from build123d import *

# Parameters (mm, degrees)
ESQUISSE1_R        = 3.5
ESQUISSE1_R_2      = 1.45
BOSS_EXTRU_1_DEPTH = 5


with BuildPart() as part:
    # Esquisse1 → Boss.-Extru.1 (new body)
    with BuildSketch(Plane.XY):
        with BuildLine():
            Line((-23.520309347, 11.085383373), (-24.358908183, 11.706502475))
            ThreePointArc((-24.358908183, 11.706502475), (-24.845678879, 12.118284674), (-25.260449538, 12.602511471))
            ThreePointArc((-25.260449538, 12.602511471), (-32.357200459, 11.85890316), (-28.166092976, 6.083832163))
            ThreePointArc((-28.166092976, 6.083832163), (-26.925251175, 6.018420638), (-25.765053202, 5.573552451))
            ThreePointArc((-25.765053202, 5.573552451), (-23.38866031, 3.221956107), (-22.477205459, 0.005358743))
            ThreePointArc((-22.477205459, 0.005358743), (-22.840333933, -2.118823087), (-23.958742219, -3.960879992))
            ThreePointArc((-23.958742219, -3.960879992), (-24.504417424, -4.651802838), (-24.955377519, -5.407958113))
            ThreePointArc((-24.955377519, -5.407958113), (-25.122929262, -5.539522919), (-25.331723523, -5.497240048))
            add(Edge.make_bspline(
                [(-27.707778762, -5.50497209), (-27.463755153, -5.421858651), (-27.208964141, -5.35321212), (-26.847281922, -5.290646334), (-26.755999287, -5.277514723), (-26.472348923, -5.247412771), (-26.276940328, -5.237520804), (-25.988433148, -5.260972525), (-25.921846007, -5.267964485), (-25.794475247, -5.289589568), (-25.737903956, -5.299827616), (-25.600175401, -5.340785914), (-25.51525962, -5.375688947), (-25.386655187, -5.458237644), (-25.359770306, -5.476681289), (-25.331723523, -5.497240048)],
                knots=[0, 0, 0, 0, 0.401379624, 0.401379624, 0.532597126, 0.532597126, 0.795032129, 0.795032129, 0.872293172, 0.872293172, 0.929035383, 0.929035383, 0.985777595, 0.985777595, 1, 1, 1, 1], degree=3))
            ThreePointArc((-27.707778762, -5.50497209), (-27.801973044, -5.564338041), (-27.859240924, -5.659822431))
            ThreePointArc((-27.859240924, -5.659822431), (-27.97528469, -6.057416591), (-28.073587363, -6.459764521))
            ThreePointArc((-28.073587363, -6.459764521), (-28.071734795, -6.57109038), (-28.019843727, -6.669600257))
            add(Edge.make_bspline(
                [(-25.965992802, -7.864336487), (-26.163909603, -7.885982848), (-26.294618647, -7.863685821), (-26.490123672, -7.810689646), (-26.569333075, -7.776803309), (-26.723621302, -7.70842793), (-26.794279204, -7.672573545), (-27.014611477, -7.551431096), (-27.148381506, -7.461400071), (-27.399282552, -7.274477346), (-27.514428456, -7.1774816), (-27.765918403, -6.946352168), (-27.896967937, -6.810004535), (-28.019843727, -6.669600257)],
                knots=[0, 0, 0, 0, 0.081187854, 0.081187854, 0.177126147, 0.177126147, 0.27306444, 0.27306444, 0.491378598, 0.491378598, 0.709692757, 0.709692757, 1, 1, 1, 1], degree=3))
            ThreePointArc((-25.965992802, -7.864336487), (-25.764030643, -7.932116803), (-25.68471018, -8.12983162))
            ThreePointArc((-25.68471018, -8.12983162), (-25.693544809, -8.474793397), (-25.684712274, -8.819755228))
            ThreePointArc((-25.684712274, -8.819755228), (-25.764033937, -9.017469563), (-25.965996507, -9.085248653))
            add(Edge.make_bspline(
                [(-28.019854683, -10.279972417), (-27.850080758, -10.085982263), (-27.663748533, -9.899137116), (-27.381805435, -9.664112445), (-27.309318159, -9.607098819), (-27.078720715, -9.439204582), (-26.914437891, -9.332933591), (-26.652857483, -9.208989788), (-26.591695348, -9.181751432), (-26.470576489, -9.136793922), (-26.416465288, -9.117374686), (-26.2767097, -9.083981334), (-26.185718951, -9.071750358), (-26.033069896, -9.078937415), (-26.000565097, -9.081467639), (-25.965996507, -9.085248653)],
                knots=[0, 0, 0, 0, 0.401379627, 0.401379627, 0.532597128, 0.532597128, 0.79503213, 0.79503213, 0.872293173, 0.872293173, 0.929035387, 0.929035387, 0.985777601, 0.985777601, 1, 1, 1, 1], degree=3))
            ThreePointArc((-28.019854683, -10.279972417), (-28.071746349, -10.37848198), (-28.073599593, -10.489807828))
            ThreePointArc((-28.073599593, -10.489807828), (-27.975299362, -10.892156354), (-27.85925801, -11.289751218))
            ThreePointArc((-27.85925801, -11.289751218), (-27.801990645, -11.385236021), (-27.707796615, -11.444602537))
            add(Edge.make_bspline(
                [(-25.331741596, -11.452348942), (-25.492319392, -11.570053641), (-25.616665259, -11.616098371), (-25.812475663, -11.66795485), (-25.898016186, -11.678213122), (-26.065821398, -11.696142421), (-26.144940129, -11.700420563), (-26.396324695, -11.705674262), (-26.557188449, -11.694590122), (-26.867936486, -11.658160819), (-27.016153634, -11.631732992), (-27.349515039, -11.557314005), (-27.531181086, -11.504758257), (-27.707796615, -11.444602537)],
                knots=[0, 0, 0, 0, 0.081187854, 0.081187854, 0.177126146, 0.177126146, 0.273064438, 0.273064438, 0.491378592, 0.491378592, 0.709692747, 0.709692747, 1, 1, 1, 1], degree=3))
            ThreePointArc((-25.331741596, -11.452348942), (-25.122947078, -11.410067338), (-24.955396133, -11.541633161))
            ThreePointArc((-24.955396133, -11.541633161), (-24.790566257, -11.844796137), (-24.610436143, -12.139125579))
            ThreePointArc((-24.610436143, -12.139125579), (-24.58027355, -12.350012048), (-24.721288721, -12.509691746))
            add(Edge.make_bspline(
                [(-25.902620196, -14.571281964), (-25.852586741, -14.318394602), (-25.784640874, -14.063415847), (-25.657983326, -13.718906965), (-25.623714317, -13.633288078), (-25.50795819, -13.372588681), (-25.418820586, -13.19841389), (-25.254257211, -12.960285204), (-25.214908427, -12.906115029), (-25.132495175, -12.806621255), (-25.095343118, -12.762748102), (-24.991007907, -12.663950818), (-24.918323098, -12.607863109), (-24.78253161, -12.537762753), (-24.753116511, -12.52370159), (-24.721288721, -12.509691746)],
                knots=[0, 0, 0, 0, 0.401379624, 0.401379624, 0.532597126, 0.532597126, 0.795032129, 0.795032129, 0.872293171, 0.872293171, 0.929035385, 0.929035385, 0.985777599, 0.985777599, 1, 1, 1, 1], degree=3))
            ThreePointArc((-25.902620196, -14.571281964), (-25.898304915, -14.682539581), (-25.844246948, -14.779877216))
            ThreePointArc((-25.844246948, -14.779877216), (-25.557942188, -15.079171145), (-25.258649996, -15.365477722))
            ThreePointArc((-25.258649996, -15.365477722), (-25.16131269, -15.41953628), (-25.0500551, -15.423852235))
            add(Edge.make_bspline(
                [(-22.988457711, -14.242533274), (-23.068669813, -14.424757432), (-23.153334128, -14.526806272), (-23.296982674, -14.669620503), (-23.365933805, -14.72127469), (-23.502292735, -14.820704525), (-23.568672495, -14.863968871), (-23.783751076, -14.994210996), (-23.928605252, -15.065043729), (-24.215935615, -15.188869049), (-24.357509352, -15.240090455), (-24.683418279, -15.342322416), (-24.867023546, -15.387640821), (-25.0500551, -15.423852235)],
                knots=[0, 0, 0, 0, 0.081187854, 0.081187854, 0.177126148, 0.177126148, 0.273064442, 0.273064442, 0.49137861, 0.49137861, 0.709692777, 0.709692777, 1, 1, 1, 1], degree=3))
            ThreePointArc((-22.988457711, -14.242533274), (-22.828777157, -14.101519072), (-22.617890871, -14.131682944))
            ThreePointArc((-22.617890871, -14.131682944), (-22.323562523, -14.311814845), (-22.020400547, -14.476646561))
            ThreePointArc((-22.020400547, -14.476646561), (-21.88883574, -14.644198304), (-21.931118612, -14.852992566))
            add(Edge.make_bspline(
                [(-21.92338657, -17.229047804), (-22.006500009, -16.985024196), (-22.075146539, -16.730233184), (-22.137712326, -16.368550965), (-22.150843937, -16.27726833), (-22.180945889, -15.993617965), (-22.190837855, -15.798209371), (-22.167386135, -15.509702191), (-22.160394175, -15.44311505), (-22.138769092, -15.315744289), (-22.128531044, -15.259172998), (-22.087572745, -15.121444441), (-22.052669711, -15.036528659), (-21.970121013, -14.907924226), (-21.951677369, -14.881039346), (-21.931118612, -14.852992566)],
                knots=[0, 0, 0, 0, 0.401379624, 0.401379624, 0.532597126, 0.532597126, 0.795032129, 0.795032129, 0.872293171, 0.872293171, 0.929035384, 0.929035384, 0.985777596, 0.985777596, 1, 1, 1, 1], degree=3))
            ThreePointArc((-21.92338657, -17.229047804), (-21.864020619, -17.323242086), (-21.768536229, -17.380509967))
            ThreePointArc((-21.768536229, -17.380509967), (-21.370942069, -17.496553733), (-20.96859414, -17.594856406))
            ThreePointArc((-20.96859414, -17.594856406), (-20.85726828, -17.593003837), (-20.758758403, -17.541112769))
            add(Edge.make_bspline(
                [(-19.564022173, -15.487261844), (-19.542375812, -15.685178645), (-19.564672839, -15.815887691), (-19.617669014, -16.011392715), (-19.651555352, -16.090602119), (-19.719930731, -16.244890347), (-19.755785117, -16.31554825), (-19.87692757, -16.535880531), (-19.9669586, -16.669650565), (-20.153881335, -16.920551621), (-20.250877086, -17.035697529), (-20.482006514, -17.287187467), (-20.618354136, -17.418236989), (-20.758758403, -17.541112769)],
                knots=[0, 0, 0, 0, 0.081187854, 0.081187854, 0.177126148, 0.177126148, 0.273064442, 0.273064442, 0.491378611, 0.491378611, 0.70969278, 0.70969278, 1, 1, 1, 1], degree=3))
            ThreePointArc((-19.564022173, -15.487261844), (-19.496241857, -15.285299686), (-19.29852704, -15.205979223))
            ThreePointArc((-19.29852704, -15.205979223), (-18.953565263, -15.214813851), (-18.608603432, -15.205981317))
            ThreePointArc((-18.608603432, -15.205981317), (-18.410889097, -15.285302979), (-18.343110007, -15.48726555))
            add(Edge.make_bspline(
                [(-17.148386243, -17.541123726), (-17.342376397, -17.3713498), (-17.529221544, -17.185017576), (-17.764246214, -16.903074479), (-17.82125984, -16.830587203), (-17.989154077, -16.599989758), (-18.095425068, -16.435706934), (-18.219368872, -16.174126527), (-18.246607228, -16.112964392), (-18.291564738, -15.991845532), (-18.310983975, -15.93773433), (-18.344377327, -15.797978738), (-18.356608302, -15.706987985), (-18.349421244, -15.554338929), (-18.34689102, -15.521834135), (-18.343110007, -15.48726555)],
                knots=[0, 0, 0, 0, 0.401379626, 0.401379626, 0.532597128, 0.532597128, 0.79503213, 0.79503213, 0.872293172, 0.872293172, 0.929035388, 0.929035388, 0.985777604, 0.985777604, 1, 1, 1, 1], degree=3))
            ThreePointArc((-17.148386243, -17.541123726), (-17.04987668, -17.593015392), (-16.938550832, -17.594868636))
            ThreePointArc((-16.938550832, -17.594868636), (-16.536202306, -17.496568405), (-16.138607442, -17.380527052))
            ThreePointArc((-16.138607442, -17.380527052), (-16.043122704, -17.323259752), (-15.983756182, -17.22906583))
            add(Edge.make_bspline(
                [(-15.976009718, -14.853010638), (-15.858305019, -15.013588435), (-15.812260288, -15.137934302), (-15.76040381, -15.333744708), (-15.750145537, -15.419285233), (-15.732216239, -15.587090447), (-15.727938096, -15.666209179), (-15.722684398, -15.917593753), (-15.733768539, -16.078457512), (-15.770197846, -16.38920556), (-15.796625675, -16.537422713), (-15.871044662, -16.870784108), (-15.923600407, -17.052450142), (-15.983756182, -17.22906583)],
                knots=[0, 0, 0, 0, 0.081187854, 0.081187854, 0.177126148, 0.177126148, 0.273064442, 0.273064442, 0.491378605, 0.491378605, 0.709692768, 0.709692768, 1, 1, 1, 1], degree=3))
            ThreePointArc((-15.976009718, -14.853010638), (-16.018291322, -14.64421612), (-15.886725499, -14.476665176))
            ThreePointArc((-15.886725499, -14.476665176), (-15.583562523, -14.3118353), (-15.289233081, -14.131705185))
            ThreePointArc((-15.289233081, -14.131705185), (-14.630974378, -13.646175845), (-14.036377119, -13.084484329))
            ThreePointArc((-14.036377119, -13.084484329), (-11.382823106, -11.204809867), (-8.204887511, -10.515425843))
            Line((-8.204887511, -10.515425843), (17.04643759, -10.514813851))
            ThreePointArc((17.04643759, -10.514813851), (18.255496355, -10.99583891), (18.803660163, -12.175976463))
            Line((18.803660163, -12.175976463), (18.803660163, -14.514813851))
            Line((18.803660163, -14.514813851), (31.285246412, -14.514813851))
            Line((31.285246412, -14.514813851), (31.285258645, -10.483748772))
            ThreePointArc((31.285258645, -10.483748772), (30.693026835, -8.420856178), (29.166459934, -6.912261511))
            Line((29.166459934, -6.912261511), (22.428792847, -3.022240342))
            ThreePointArc((22.428792847, -3.022240342), (14.240952746, -0.032887143), (5.524515127, -0.006939391))
            Line((5.524515127, -0.006939391), (-9.47465467, -2.651398118))
            ThreePointArc((-9.47465467, -2.651398118), (-13.371139001, -1.975728488), (-15.913565792, 1.053328395))
            ThreePointArc((-15.913565792, 1.053328395), (-18.956552603, 6.645913075), (-23.520309347, 11.085383373))
        make_face()
        with Locations((-18.953544809, -8.474813851)):
            Circle(ESQUISSE1_R, mode=Mode.SUBTRACT)
        with Locations((-28.594110039, 10.181539009)):
            Circle(ESQUISSE1_R_2, mode=Mode.SUBTRACT)
    extrude(amount=BOSS_EXTRU_1_DEPTH)


solid = part.part
Source: CAD feature listing. Evaluate the final solid. Frame: model axes, mm. A direction names the side the tool comes from. Round coordinates to 2 decimals unless told otherwise and drop trailing zeros. Order: outer loops, then holes, each group sorted by start corner. A loop starts at its lowest first (then second) coordinate and runs counter-clockwise, first axis right, second up. Notation, with made-up numbers: (14, -20.5) - (39, -20.5) arc R17 ccw to (39, 0.5) - close; hole circle Ø4 at (-9, 11). An arc over 180 degrees is marked (long way). Use a Markdown table: item, result. Add a question column.
1. Section query B-B (x = 1). Return the cut outline in (y, z).
2. Line query: probe 1 along Y at (x, z) = (-25.5, 1.85); probe 2 along Y at (x, z) = (-21.5, 3.4); probe 3 along Y at (x, z) = (-24, 0.7). Output: solid intervals per line, ascending.
3. First-contact query: pin 1 (3 mm diameter, centred on y = -10.5, z = 1.5, fed in from -X); pin 2 (1 mm diameter, centred on y = -11.5, z = 4.5, fed in from -X); pin 3 (0.7 mm diameter, centred on y = -13.5, z = 2.5, fed in from -X). Flat tips, straight axial feed; report the tip coordinate or a pass-through.
4. Mould query, pull axis X, two halves, no side actions, for faces 6 (the cylindrical face through (-23.41, 3.26, 2.46)), 7 (the cylindrical face through (-18.9, 6.57, 2.46)), 8 (the cylindrical face through (-11.42, -11.22, 2.46)), 9 (the flat face through (-3, -4, 5)). Classes: +X half, -X half, draft (parallel to the pull), parting line (faces both ways), or undercut.
5. Section query A-A (y = 3). Return the cut outline in (x, z), then the cut area to 3 significant figures.
6. Section query C-C (z = 1.1). Give the number of separate pieces and of enclosed holes in the cut face, then the cut area to 3 significant figures.
7. Set-up query: faces 1 (the cylindrical face through (18.24, -10.98, 2.46)), 2 (the flat face through (-1.87, -1.31, 2.46)), 3 (the cylindrical face through (-26.94, 6.02, 2.46)), 4 (the flat face through (25, -14.515, 2)), 5 (the cylindrical face through (-22.83, -2.09, 2.46)). Return all of +Z, -Z, +X, -X, +Y, -Y with unobstructed straight access to the full face (end or side cutting, diameter ignored); none if empty.
Derived:
| question | item | result |
|---|---|---|
| 1 | outline | (-10.52, 0) - (-0.8, 0) - (-0.8, 5) - (-10.52, 5) - close |
| 2 | probe 1 | -15.14 to -13.37, -11.56 to -5.39, 5.41 to 12.9 |
| 2 | probe 2 | -17.46 to -10.88, -6.07 to 9.44 |
| 2 | probe 3 | -15.1 to -4.01, 4.09 to 11.44 |
| 3 | pin 1 | x = -28.08 |
| 3 | pin 2 | x = -27.95 |
| 3 | pin 3 | x = -25.71 |
| 4 | face 6 | -X half |
| 4 | face 7 | +X half |
| 4 | face 8 | undercut |
| 4 | face 9 | draft |
| 5 | outline | (-23.26, 0) - (-16.73, 0) - (-16.73, 5) - (-23.26, 5) - close |
| 5 | area | 32.7 mm2 |
| 6 | separate pieces | 1 |
| 6 | enclosed holes | 2 |
| 6 | area | 693 mm2 |
| 7 | face 1 | +Z, -Z, -Y |
| 7 | face 2 | +Z, -Z, +Y |
| 7 | face 3 | +Z, -Z |
| 7 | face 4 | +Z, -Z, +X, -Y |
| 7 | face 5 | +Z, -Z, -X |
